```python
from build123d import *

# Parameters (mm, degrees)
SALIENTE_EXTRUIR1_DEPTH = 13.8
CROQUIS3_R              = 1.5
CORTAR_EXTRUIR1_DEPTH   = 10
CROQUIS3_3_R            = 2.9
CROQUIS3_3_R_2          = 1.5
CORTAR_EXTRUIR2_DEPTH   = 7.5
REDONDEO1_R             = 1
REDONDEO2_R             = 2
REDONDEO3_R             = 1.5


with BuildPart() as part:
    # Croquis1 → Saliente-Extruir1 (new body)
    with BuildSketch(Plane(origin=(0, 0, 0), x_dir=(0, 0, -1), z_dir=(1, 0, 0))):
        Polygon((-6, 0), (6, 0), (6, -10), (14.3, -10), (14.3, -7.5), (11.5, -7.5), (8.25, 2), (-8.25, 2), (-11.5, -7.5), (-14.3, -7.5), (-14.3, -10), (-6, -10), align=None)
    extrude(amount=SALIENTE_EXTRUIR1_DEPTH)

    # Croquis3 → Cortar-Extruir1 (cut)
    with BuildSketch(Plane(origin=(0, 0, 0), x_dir=(1, 0, 0), z_dir=(0, 1, 0))):
        with Locations(Location((6.9, -11.5, 0), (0, 0, 270))):
            Circle(CROQUIS3_R)
        with Locations(Location((6.9, 11.5, 0), (0, 0, 270))):
            Circle(CROQUIS3_R)
    extrude(amount=-CORTAR_EXTRUIR1_DEPTH, mode=Mode.SUBTRACT)

    # Croquis3<3> → Cortar-Extruir2 (cut)
    # profile 1 of 2: a face of its own
    with BuildSketch(Plane(origin=(0, 0, 0), x_dir=(1, 0, 0), z_dir=(0, 1, 0))):
        with Locations((6.9, -11.5)):
            Circle(CROQUIS3_3_R)
        with Locations(Location((6.9, -11.5, 0), (0, 0, 270))):
            Circle(CROQUIS3_3_R_2, mode=Mode.SUBTRACT)
    # profile 2 of 2: a face of its own
    with BuildSketch(Plane(origin=(0, 0, 0), x_dir=(1, 0, 0), z_dir=(0, 1, 0))):
        with Locations((6.9, 11.5)):
            Circle(CROQUIS3_3_R)
        with Locations(Location((6.9, 11.5, 0), (0, 0, 270))):
            Circle(CROQUIS3_3_R_2, mode=Mode.SUBTRACT)
    extrude(amount=-CORTAR_EXTRUIR2_DEPTH, mode=Mode.SUBTRACT)

    # Redondeo1
    redondeo1_edges = [part.edges().sort_by_distance(p)[0] for p in [
        (6.9, 0, -6),
        (6.9, 0, 6),
    ]]
    fillet(redondeo1_edges, radius=REDONDEO1_R)

    # Redondeo2
    redondeo2_edges = [part.edges().sort_by_distance(p)[0] for p in [
        (6.9, 2, 8.25),
        (6.9, 2, -8.25),
    ]]
    fillet(redondeo2_edges, radius=REDONDEO2_R)

    # Redondeo3
    redondeo3_edges = [part.edges().sort_by_distance(p)[0] for p in [
        (13.8, -8.75, -14.3),
        (0, -8.75, 14.3),
        (0, -8.75, -14.3),
        (13.8, -8.75, 14.3),
    ]]
    fillet(redondeo3_edges, radius=REDONDEO3_R)


solid = part.part
```
Source: CAD feature listing. Evaluate the final solid. Frame: model axes, mm. A direction names the side the tool comes from. Coordinates: 2 decimals unless noted, no trailing zeros. Loops run counter-clockwise (first coordinate to the right, second up) from the corner with the lowest first, then second, coordinate; pieces in that order, holes last. Notation, with made-up numbers: M 31,3 L 90,3 A31 ccw 90,32 Z; hole C 48.25,-36.5 d4. An arc over 180 degrees is marked long. Use CSV: the item, a comma, the result in double quotes.
(1) Contact query for flat-ended pins moving along their axis: pin 1 (1 mm diameter, centred on x = 8.5, y = 0.5, fed in from +Z); pin 2 (7 mm diameter, centred on x = 5.5, y = -6.5, fed in from -Z); pin 3 (2 mm diameter, centred on x = 10, y = -3, fed in from -Z); pin 4 (5 mm diameter, centred on x = 9.5, z = -1, fed in from -Y). Output: stop coordinate, or through.
Answers follow:
pin 1,"z = 8.93"
pin 2,"z = -14.3"
pin 3,"z = -10.3"
pin 4,"y = 0"
(2) Line query: line 1 (Z direction, x = 6.9, y = -8.75); line 2 (X direction, y = -8.7, z = 11.5); line 3 (Z direction, x = 7.75, y = -8.75). Output: solid intervals per line, ascending. Write a range as [from, to].
Answers follow:
line 1,"[-14.3, -13], [-10, -6], [6, 10], [13, 14.3]"
line 2,"[0, 5.4], [8.4, 13.8]"
line 3,"[-14.3, -12.74], [-10.26, -6], [6, 10.26], [12.74, 14.3]"
(3) Cut plane B-B on x = 6.9. Return loops of the section in (y, z).
Answers follow:
outline,"M -10,-14.3 L -7.5,-14.3 L -7.5,-13 L -10,-13 Z; M -10,-10 L -7.5,-10 L -7.5,-8.6 L 0,-8.6 L 0,-8.93 L 0.65,-8.71 A2 ccw 2,-6.82 L 2,6.82 A2 ccw 0.65,8.71 L 0,8.93 L 0,8.6 L -7.5,8.6 L -7.5,10 L -10,10 L -10,6 L -1,6 A1 cw 0,5 L 0,-5 A1 cw -1,-6 L -10,-6 Z; M -10,13 L -7.5,13 L -7.5,14.3 L -10,14.3 Z"
(4) Cut plane A-A on y = -8.75. Return loops of the section in (x, z).
Answers follow:
outline,"M 0,-12.8 A1.5 ccw 1.5,-14.3 L 12.3,-14.3 A1.5 ccw 13.8,-12.8 L 13.8,-6 L 0,-6 Z; M 0,6 L 13.8,6 L 13.8,12.8 A1.5 ccw 12.3,14.3 L 1.5,14.3 A1.5 ccw 0,12.8 Z; hole C 6.9,-11.5 d3; hole C 6.9,11.5 d3"
(5) Draft query along Z for faces 1 (the face through (7, -10, 9)), 2 (the face through (13.35, -8.77, 13.87)), 3 (the face through (6.997, -0.285, -5.699)). Return one class per face: pulls with the +Z half, pulls with the -Z half, needs draft (parallel to the pull), parting line crosses it, or undercut.
Answers follow:
face 1,"needs draft"
face 2,"pulls with the +Z half"
face 3,"undercut"
(6) Cut plane D-D on x = 2.5. Return loops of the section in (y, z), and give its area (3 significant figures).
Answers follow:
outline,"M -10,-14.3 L -7.5,-14.3 L -7.5,-11.5 L 0.65,-8.71 A2 ccw 2,-6.82 L 2,6.82 A2 ccw 0.65,8.71 L -7.5,11.5 L -7.5,14.3 L -10,14.3 L -10,6 L -1,6 A1 cw 0,5 L 0,-5 A1 cw -1,-6 L -10,-6 Z"
area,"139 mm²"
(7) Cut plane C-C on z = -10.5. Return loops of the section in (x, y), and give its area (3 significant figures).
Answers follow:
outline,"M 0,-10 L 5.78,-10 L 5.78,-7.5 L 4.18,-7.5 L 4.18,-4.58 L 0,-4.58 Z; M 8.02,-10 L 13.8,-10 L 13.8,-4.58 L 9.62,-4.58 L 9.62,-7.5 L 8.02,-7.5 Z"
area,"53.3 mm²"
(8) Reachability of faces 4 (the face through (7, 0, 0)), 5 (the face through (7, -4.5, 8.6)), 6 (the face through (6.997, 1.617, -7.998)) from +Z, -Z, +X, -X, +Y, -Y: full face, straight path, thin tool, end or side. Return the list, or none.
Answers follow:
face 4,"+X, -X, -Y"
face 5,"+Z"
face 6,"-Z, +X, -X, +Y"
